Input: part model. Units: mm. Frame: model coordinates. Round coordinates to 2 decimals unless told otherwise and drop trailing zeros. Loops run counter-clockwise (first coordinate to the right, second up) from the corner with the lowest first, then second, coordinate; pieces in that order, holes last. Notation, with made-up numbers: (13.5, 72.5) - (65.5, 72.5) arc R14 ccw to (65.5, 87.5) - close; hole circle Ø11 at (-32, -37). An arc over 180 degrees is marked (long way). Use CSV: the item, a comma, the result in double quotes. Start each with the question number.
1. Cut plane B-B (x = -7.5). Return loops of the section in (y, z), and give its area (3 significant figures).
2. Cut plane A-A (z = -121.5). Return loops of the section in (x, y), and give its area (3 significant figures).
3. Cut plane C-C (y = 3.5). Give the number of separate pieces and of enclosed holes in the cut face, and give its area (3 significant figures).
4. Pin query (flat end, axial travel): P1, Ø1.9, axis at x = 6, y = 4, coming from the +Z side; P2, Ø3, axis at x = -4.5, y = 3.5, coming from the -Z side; P3, Ø3, axis at x = -10, y = 5, coming from the +Z side; P4, Ø1.8, axis at x = 19.34, z = -180.66, coming from the -Y side. Return the tip coordinate at first contact, or that it passes through.
5. Cut plane D-D (z = -87.7). Return loops of the section in (x, y), and give its area (3 significant figures).
6. Material intervals for probe 1 along X at (y, z) = (3.25, -199.5); probe 2 along Z at (x, y) = (19, 2.5); probe 3 along Z at (x, y) = (12, 3), sorted ascending. Write a range as from..to.
```python
from build123d import *

# Parameters (mm, degrees)
BOSS_EXTRUDE1_DEPTH     = 6.35
SKETCH2_R               = 2.6
CUT_EXTRUDE1_DEPTH      = 238.676928834
ESQUISSE3_R             = 21
ENL_V_MAT_EXTRU_2_DEPTH = 238.676928834
ESQUISSE7_R             = 1.5
ENL_V_MAT_EXTRU_3_DEPTH = 238.676928834
CUT_EXTRUDE2_DEPTH      = 238.676928834
SKETCH5_R               = 1.625
CUT_EXTRUDE3_DEPTH      = 238.676928834
CUT_EXTRUDE5_DEPTH      = 238.676928834


with BuildPart() as part:
    # Sketch1 → Boss-Extrude1 (new body)
    with BuildSketch(Plane(origin=(0, 0, 0), x_dir=(1, 0, 0), z_dir=(0, 1, 0))):
        with BuildLine():
            Line((27.5, 0), (34.975254116, 198.684097441))
            ThreePointArc((34.975254116, 198.684097441), (0, 235), (-34.975254116, 198.684097441))
            Line((-34.975254116, 198.684097441), (-27.5, 0))
            ThreePointArc((-27.5, 0), (0, -27.5), (27.5, 0))
        make_face()
    extrude(amount=BOSS_EXTRUDE1_DEPTH)

    # Sketch2 → Cut-Extrude1 (cut, through all)
    with BuildSketch(Plane(origin=(0, 6.35, 0), x_dir=(1, 0, 0), z_dir=(0, 1, 0))):
        with Locations(Location((0, 0, 0), (0, 0, 270))):
            Circle(SKETCH2_R)
    extrude(amount=-CUT_EXTRUDE1_DEPTH, mode=Mode.SUBTRACT)

    # Esquisse3 → Enlèv. mat.-Extru.2 (cut, through all)
    with BuildSketch(Plane(origin=(0, 6.35, 0), x_dir=(1, 0, 0), z_dir=(0, 1, 0))):
        with Locations(Location((0, 200, 0), (0, 0, 270))):
            Circle(ESQUISSE3_R)
    extrude(amount=-ENL_V_MAT_EXTRU_2_DEPTH, mode=Mode.SUBTRACT)

    # Esquisse7 → Enlèv. mat.-Extru.3 (cut, through all)
    with BuildSketch(Plane(origin=(0, 6.35, 0), x_dir=(1, 0, 0), z_dir=(0, 1, 0))):
        with Locations(Location((-19.339370465, 219.339370465, 0), (0, 0, 270))):
            Circle(ESQUISSE7_R)
        with Locations(Location((19.339370465, 219.339370465, 0), (0, 0, 270))):
            Circle(ESQUISSE7_R)
        with Locations(Location((19.339370465, 180.660629535, 0), (0, 0, 270))):
            Circle(ESQUISSE7_R)
        with Locations(Location((-19.339370465, 180.660629535, 0), (0, 0, 270))):
            Circle(ESQUISSE7_R)
    extrude(amount=-ENL_V_MAT_EXTRU_3_DEPTH, mode=Mode.SUBTRACT)

    # Sketch3 → Cut-Extrude2 (cut, through all)
    with BuildSketch(Plane(origin=(0, 6.35, 0), x_dir=(1, 0, 0), z_dir=(0, 1, 0))):
        Polygon((21.15, 145.828069991), (21.15, 111.871930009), (16.978069991, 107.7), (-16.978069991, 107.7), (-21.15, 111.871930009), (-21.15, 145.828069991), (-16.978069991, 150), (16.978069991, 150), align=None)
    extrude(amount=-CUT_EXTRUDE2_DEPTH, mode=Mode.SUBTRACT)

    # Sketch5 → Cut-Extrude3 (cut, through all)
    with BuildSketch(Plane(origin=(0, 6.35, 0), x_dir=(1, 0, 0), z_dir=(0, 1, 0))):
        with Locations(Location((-27.256476824, 142.340455159, 0), (0, 0, 270))):
            Circle(SKETCH5_R)
        with Locations(Location((-26.241351992, 115.359544841, 0), (0, 0, 270))):
            Circle(SKETCH5_R)
    cut_extrude3 = extrude(amount=-CUT_EXTRUDE3_DEPTH, mode=Mode.SUBTRACT)

    # Mirror1: Cut-Extrude3 across plane
    add(cut_extrude3.mirror(Plane(origin=(0, 0, 0), x_dir=(0, 0, 1), z_dir=(1, 0, 0))), mode=Mode.SUBTRACT)

    # Sketch8 → Cut-Extrude5 (cut, through all)
    with BuildSketch(Plane(origin=(0, 6.35, 0), x_dir=(1, 0, 0), z_dir=(0, 1, 0))):
        with BuildLine():
            Line((-12.749738424, 90.764177772), (17.892039301, 65.052673385))
            ThreePointArc((17.892039301, 65.052673385), (18.385066635, 59.417345174), (12.749738424, 58.92431784))
            Line((12.749738424, 58.92431784), (-17.892039301, 84.635822228))
            ThreePointArc((-17.892039301, 84.635822228), (-18.385066635, 90.271150439), (-12.749738424, 90.764177772))
        make_face()
    extrude(amount=-CUT_EXTRUDE5_DEPTH, mode=Mode.SUBTRACT)


solid = part.part
```
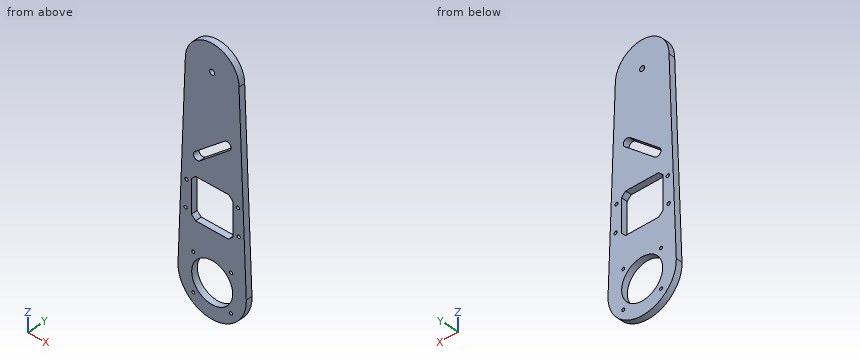
Established:
1,outline,"(0, -234.19) - (6.35, -234.19) - (6.35, -219.62) - (0, -219.62) - close; (0, -180.38) - (6.35, -180.38) - (6.35, -150) - (0, -150) - close; (0, -107.7) - (6.35, -107.7) - (6.35, -86.36) - (0, -86.36) - close; (0, -75.92) - (6.35, -75.92) - (6.35, 26.46) - (0, 26.46) - close"
1,area,"1,070 mm2"
2,outline,"(-32.07, 0) - (-21.15, 0) - (-21.15, 6.35) - (-32.07, 6.35) - close; (21.15, 0) - (32.07, 0) - (32.07, 6.35) - (21.15, 6.35) - close"
2,area,"139 mm2"
3,separate pieces,"1"
3,enclosed holes,"12"
3,area,"12,000 mm2"
4,P1,"stops at z = 27.03"
4,P2,"stops at z = -234.87"
4,P3,"stops at z = 26.15"
4,P4,"passes through"
5,outline,"(-30.8, 0) - (-19.32, 0) - (-19.32, 6.35) - (-30.8, 6.35) - close; (-9.1, 0) - (30.8, 0) - (30.8, 6.35) - (-9.1, 6.35) - close"
5,area,"326 mm2"
6,probe 1,"x = -35..-20.99, 20.99..35"
6,probe 2,"z = -229.39..-220.8, -217.88..-208.94, -191.06..-182.12, -179.2..-147.98, -109.72..-63.56, -60.42..19.88"
6,probe 3,"z = -232.88..-217.23, -182.77..-150, -107.7..-70, -59.55..24.74"
